```python
from build123d import *
from OCP.BRepFilletAPI import BRepFilletAPI_MakeFillet

# Parameters (mm, degrees)
BOSS_EXTRUDE1_DEPTH      = 30.1625
BOSS_EXTRUDE1_DEPTH_BACK = 30.1625
SKETCH1_R                = 3.96875
SKETCH2_W                = 53.975
SKETCH2_H                = 127
CUT_EXTRUDE1_DEPTH       = 138.343982508
SKETCH3_R                = 9.525
BOSS_EXTRUDE2_DEPTH      = 63.5
FILLET5_R1               = 6.35
FILLET5_R2               = 2.54


with BuildPart() as part:
    # Sketch1 → Boss-Extrude1 (new, two sides: drawn at the far end of the back side and taken through both)
    with BuildSketch(Plane(origin=(0, 0, 0), x_dir=(0, 0, -1), z_dir=(1, 0, 0)).offset(-BOSS_EXTRUDE1_DEPTH_BACK)):
        with BuildLine():
            Line((-66.675, 107.95), (-34.925, 107.95))
            Line((-34.925, 107.95), (-34.925, 95.25))
            ThreePointArc((-34.925, 95.25), (-23.848499799, 47.977772084), (7.075086505, 10.546712803))
            ThreePointArc((7.075086505, 10.546712803), (10.546712803, -7.075086505), (-7.075086505, -10.546712803))
            ThreePointArc((-7.075086505, -10.546712803), (-50.749935163, 34.535310409), (-66.675, 95.25))
            Line((-66.675, 95.25), (-66.675, 107.95))
        make_face()
        Circle(SKETCH1_R, mode=Mode.SUBTRACT)
    extrude(amount=BOSS_EXTRUDE1_DEPTH + BOSS_EXTRUDE1_DEPTH_BACK)

    # Sketch2 → Cut-Extrude1 (cut, through all)
    with BuildSketch(Plane.XY.offset(66.675)):
        with Locations((0, 31.75)):
            Rectangle(SKETCH2_W, SKETCH2_H)
    extrude(amount=-CUT_EXTRUDE1_DEPTH, mode=Mode.SUBTRACT)

    # Sketch3 → Boss-Extrude2 (add)
    with BuildSketch(Plane(origin=(0, 107.95, 0), x_dir=(1, 0, 0), z_dir=(0, 1, 0))):
        with Locations(Location((0, -50.8, 0), (0, 0, 270))):
            Circle(SKETCH3_R)
    extrude(amount=BOSS_EXTRUDE2_DEPTH)

    # Fillet5: one fillet with a radius per group of edges: ONE call of the kernel's fillet builder (fillet() takes one radius for all edges)
    fillet5_edges_1 = [part.edges().sort_by_distance(p)[0] for p in [
        (-30.1625, 107.95, 50.8),
        (30.1625, 107.95, 50.8),
    ]]
    fillet5_edges_2 = [part.edges().sort_by_distance(p)[0] for p in [
        (0, 107.95, 34.925),
        (0, 107.95, 66.675),
    ]]
    fillet5 = BRepFilletAPI_MakeFillet(part.part.solid().wrapped)
    for e in fillet5_edges_1:
        fillet5.Add(FILLET5_R1, e.wrapped)
    for e in fillet5_edges_2:
        fillet5.Add(FILLET5_R2, e.wrapped)
    add(Compound.cast(fillet5.Shape()), mode=Mode.REPLACE)


solid = part.part
```
Geometry check sheet. Reference: the model listing, model coordinates, mm. A direction names the side the tool comes from. Round coordinates to 2 decimals unless told otherwise and drop trailing zeros. Write each loop counter-clockwise with the first axis right and the second up, starting at its lowest first coordinate (ties: lowest second). Pieces come first, ordered by that corner, then holes. Notation, with made-up numbers: (32.25, 7.5) - (39.25, 7.5) arc R11 cw to (39.25, 28.5) - close; hole circle Ø8 at (-0.75, 44.25). An arc over 180 degrees is marked (long way). Write each question's results on one line, items separated by ' | '.
(1) Set-up check for faces 4 (the face through (0, 95.25, 51)), 5 (the face through (-28.25, 106.14, 50.58)), 6 (the face through (0.419, 139.256, 41.284)): record each of +Z, -Z, +X, -X, +Y, -Y from which the full face is reachable in a straight line by a thin tool's end or side.
Computed:
face 4: +Z, -Z, -Y | face 5: +Z, -Z, -X, +Y | face 6: +Y
(2) Sectioned sample at A-A, the plane x = 0. Enter the section's corners in (y, z) (3 decimals).
Computed:
outline: (95.25, 34.925) - (105.41, 34.925) arc R2.54 ccw to (107.95, 37.465) - (107.95, 41.275) - (171.45, 41.275) - (171.45, 60.325) - (107.95, 60.325) - (107.95, 64.135) arc R2.54 ccw to (105.41, 66.675) - (95.25, 66.675) - close
(3) Sectioned sample at D-D, the plane z = 0. Enter the section's corners in (x, y).
Computed:
outline: (-30.16, -12.7) - (-26.99, -12.7) - (-26.99, -3.97) - (-30.16, -3.97) - close; (-30.16, 3.97) - (-26.99, 3.97) - (-26.99, 16.43) - (-30.16, 16.43) - close; (26.99, -12.7) - (30.16, -12.7) - (30.16, -3.97) - (26.99, -3.97) - close; (26.99, 3.97) - (30.16, 3.97) - (30.16, 16.43) - (26.99, 16.43) - close
(4) Sectioned sample at B-B, the plane y = 0. Enter the section's corners in (x, z).
Computed:
outline: (-30.16, -12.7) - (-26.99, -12.7) - (-26.99, -3.97) - (-30.16, -3.97) - close; (-30.16, 3.97) - (-26.99, 3.97) - (-26.99, 21.9) - (-30.16, 21.9) - close; (26.99, -12.7) - (30.16, -12.7) - (30.16, -3.97) - (26.99, -3.97) - close; (26.99, 3.97) - (30.16, 3.97) - (30.16, 21.9) - (26.99, 21.9) - close
(5) Sectioned sample at C-C, the plane z = 23.5. Enter the section's corners in (x, y).
Computed:
outline: (-30.16, 1.35) - (-26.99, 1.35) - (-26.99, 47.28) - (-30.16, 47.28) - close; (26.99, 1.35) - (30.16, 1.35) - (30.16, 47.28) - (26.99, 47.28) - close
(6) Thickness scan on probe 1 along Y at (x, z) = (5, 39.5); probe 2 along Y at (x, z) = (-28.35, 0); probe 3 along Z at (x, y) = (-29.05, 0). Record the ranges inside material, lowest first. Write a range as from..to.
Computed:
probe 1: y = 95.25..107.95 | probe 2: y = -12.7..-3.97, 3.97..16.43 | probe 3: z = -12.7..-3.97, 3.97..21.9
(7) Draft check along Z on faces 1 (the face through (0, 100, 66.675)), 2 (the face through (28.553, -3.874, 0.86)), 3 (the face through (26.988, 41, 28)). Enter one of: pulls with the +Z half, pulls with the -Z half, needs draft (parallel to the pull), parting line crosses it, or undercut.
Computed:
face 1: pulls with the +Z half | face 2: undercut | face 3: needs draft
(8) Depth check by flat-ended pin: pin 1 Ø10.5 at (y, z) = (0, 0) entering from -X; pin 2 Ø16 at (x, z) = (-8, 58) entering from -Y; pin 3 Ø5 at (x, y) = (12, 101.5) entering from -Z (3 decimals). Enter the tip coordinate at first touch or a pass-through.
Computed:
pin 1: stops at x = -30.16 | pin 2: stops at y = 95.25 | pin 3: stops at z = 34.925
